```python
from build123d import *

# Parameters (mm, degrees)
SKETCH1_W           = 85
SKETCH1_H           = 58
BOSS_EXTRUDE1_DEPTH = 2
SKETCH2_R           = 1
BOSS_EXTRUDE3_DEPTH = 6.5


with BuildPart() as part:
    # Sketch1 → Boss-Extrude1 (new body)
    with BuildSketch(Plane.XY):
        with Locations((-42.5, 29)):
            Rectangle(SKETCH1_W, SKETCH1_H)
    extrude(amount=BOSS_EXTRUDE1_DEPTH)

    # Sketch2 → Boss-Extrude3 (add)
    with BuildSketch(Plane.XY.offset(2)):
        with Locations((-83, 56)):
            Circle(SKETCH2_R)
        with Locations((-2, 56)):
            Circle(SKETCH2_R)
        with Locations((-83, 2)):
            Circle(SKETCH2_R)
        with Locations((-2, 2)):
            Circle(SKETCH2_R)
    extrude(amount=-BOSS_EXTRUDE3_DEPTH)


solid = part.part
```
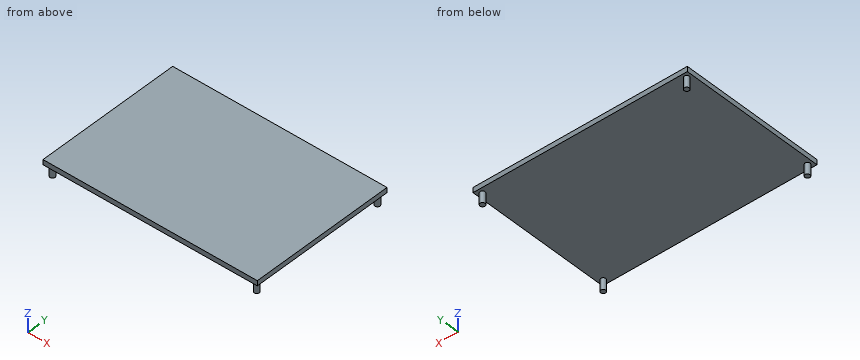
Could you check a few things on this model? Use its own coordinates, in mm. Round coordinates to 2 decimals unless told otherwise and drop trailing zeros. Write each loop counter-clockwise with the first axis right and the second up, starting at its lowest first coordinate (ties: lowest second). Pieces come first, ordered by that corner, then holes.
(1) Suppose I cut it at C-C on z = -1.75. Write out the boundary of the cut face in (x, y).
Findings below:
outline: circle Ø2 at (-83, 2); circle Ø2 at (-83, 56); circle Ø2 at (-2, 2); circle Ø2 at (-2, 56)
(2) For pin 1 (1.5 mm diameter, centred on y = 41, z = 0.5, fed in from +X); pin 2 (10 mm diameter, centred on x = -35, y = 28, fed in from -Z), each with a flat end and sliding along its axis, tell me the tip position at first contact or that it passes through.
Findings below:
pin 1: stops at x = 0
pin 2: stops at z = 0
(3) Suppose I cut it at D-D on x = -60.5. Write out the boundary of the cut face in (y, z), and give its area (3 significant figures).
Findings below:
outline: (0, 0) - (58, 0) - (58, 2) - (0, 2) - close
area: 116 mm2
(4) Suppose I cut it at B-B on y = 56. Write out the boundary of the cut face in (x, z).
Findings below:
outline: (-85, 0) - (-84, 0) - (-84, -4.5) - (-82, -4.5) - (-82, 0) - (-3, 0) - (-3, -4.5) - (-1, -4.5) - (-1, 0) - (0, 0) - (0, 2) - (-85, 2) - close
(5) Suppose I cut it at A-A on x = -83. Write out the boundary of the cut face in (y, z), and give its area (3 significant figures).
Findings below:
outline: (0, 0) - (1, 0) - (1, -4.5) - (3, -4.5) - (3, 0) - (55, 0) - (55, -4.5) - (57, -4.5) - (57, 0) - (58, 0) - (58, 2) - (0, 2) - close
area: 134 mm2
(6) If I drill on probe 1 along Z at (x, y) = (-21, 24), over which ranges is the centre line in solid material (lowest first)?
Findings below:
probe 1: z = 0 to 2
